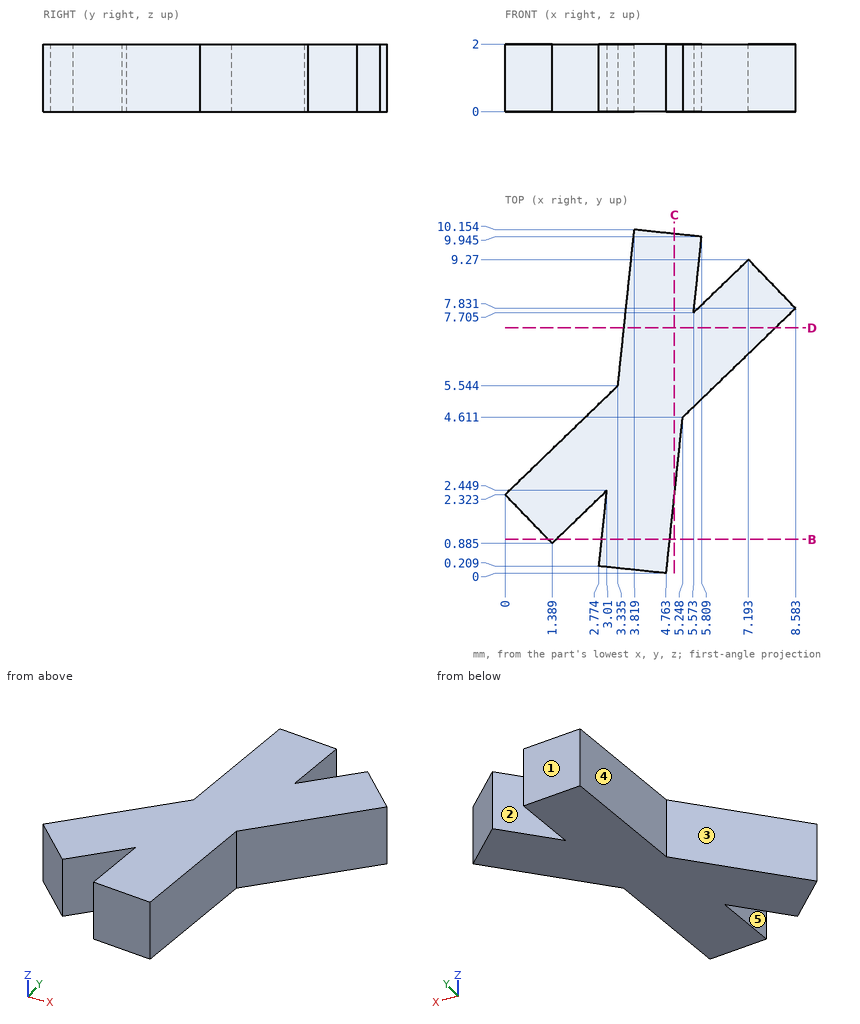
Job drawing, mm, ordinate dimensions from the low corner. One solid piece. A direction names the side the tool comes from. Give positions to 0.01 mm unless a question says otherwise; leave off trailing zeros. Order: outer loops, then holes, each group sorted by start corner. A loop starts at its lowest first (then second) coordinate and runs counter-clockwise, first axis right, second up. Notation, with made-up numbers: M 45.5,20 L 52.5,20 A16 cw 52.5,49 Z; hole C 32.5,18 d4. An arc over 180 degrees is marked long. Put each result on its own line as item: value. Start each with the question number.
(1) Band-saw the part on C-C on x = 5. Give the cut face in (y, z).
(2) Band-saw the part on B-B on y = 1. Give the cut face in (x, z).
(3) Pull direction X, two halves, no side cores. Call the marked faces 1, 2 and 3: released by +X, released by -X, zero draft, split by the parting line, or undercut.
(4) Band-saw the part on D-D on y = 7.25. Give the cut face in (x, z) (1 decimal).
(5) Pin check, flat tips, straight feed: pin 1 Ø2 at (x, y) = (2.5, 3) entering from -Z; pin 2 Ø5 at (x, y) = (7.5, 1.5) entering from -Z. Stop position of each tip, or through.
(6) Tool access for the marked faces 4 and 5: list every direction of +Z, -Z, +X, -X, +Y, -Y with a clear straight run to the whole face (end or side of a thin tool).
(7) Drill centre lines: L1, parallel to X at y = 2, z = 1 (1 decimal); L2, parallel to X at y = 9, z = 0.25 (1 decimal); L3, parallel to Y at x = 2, z = 0.4 (1 decimal). Where is each one in solid material? Low to high. Write a range as [from, to].
Results below:
1. outline: M 2.25,0 L 10.03,0 L 10.03,2 L 2.25,2 Z
2. outline: M 1.28,0 L 1.51,0 L 1.51,2 L 1.28,2 Z; M 2.86,0 L 4.87,0 L 4.87,2 L 2.86,2 Z
3. face 1: released by +X
3. face 2: undercut
3. face 3: released by -X
4. outline: M 3.5,0 L 8,0 L 8,2 L 3.5,2 Z
5. pin 1: stops at z = 0
5. pin 2: passes through
6. face 4: +Z, -Z, -X, +Y
6. face 5: +Z, -Z
7. L1: x = [0.3, 2.5], [3, 5]
7. L2: x = [3.7, 5.7], [6.9, 7.5]
7. L3: y = [1.5, 4.3]
